```python
from build123d import *

# Parameters (mm, degrees)
CROQUIS1_R              = 20
SALIENTE_EXTRUIR1_DEPTH = 10
CROQUIS2_W              = 60
CROQUIS2_H              = 45
SALIENTE_EXTRUIR2_DEPTH = 10


with BuildPart() as part:
    # Croquis1 → Saliente-Extruir1 (new body)
    with BuildSketch(Plane.XY):
        Circle(CROQUIS1_R)
    extrude(amount=SALIENTE_EXTRUIR1_DEPTH)

    # Croquis2 → Saliente-Extruir2 (add)
    with BuildSketch(Plane.XY.offset(10)):
        Rectangle(CROQUIS2_W, CROQUIS2_H)
    extrude(amount=SALIENTE_EXTRUIR2_DEPTH)


solid = part.part
```
Model file for the job. Use its own axes, mm. A direction names the side the tool comes from. Give positions to 0.01 mm unless a question says otherwise; leave off trailing zeros. Order: outer loops, then holes, each group sorted by start corner. A loop starts at its lowest first (then second) coordinate and runs counter-clockwise, first axis right, second up.
1) Saw through at B-B, the plane x = 0. Write the cut outline in (y, z).
2) 3-axis set-ups, long thin cutter, end or side, ignore diameter. For faces 1 (the flat face through (0, -22.5, 15)), 2 (the cylindrical face through (-4.336, -19.524, 4.93)): which of +Z, -Z, +X, -X, +Y, -Y reach the whole face in a straight line?
3) Saw through at C-C, the plane z = 8. Write the cut outline in (x, y), then the cut area to 3 significant figures.
4) Wall check: probe 1 along Z at (x, y) = (13.5, -20); probe 2 along X at (y, z) = (4.5, 8); probe 3 along X at (y, z) = (16.5, 6). Give the ranges that are in metal, low to high.
5) Saw through at D-D, the plane x = 22. Write the cut outline in (y, z).
6) Pin check, flat tips, straight feed: pin 1 (1.5 mm diameter, centred on x = -16, z = 8, fed in from -Y); pin 2 (5 mm diameter, centred on x = 9, z = 6.5, fed in from -Y); pin 3 (1.5 mm diameter, centred on y = 1.5, z = 9, fed in from -X). Stop position of each tip, or through.
7) Saw through at A-A, the plane y = 0. Write the cut outline in (x, z), then the cut area to 3 significant figures.
Computed:
1. outline: (-22.5, 10) - (-20, 10) - (-20, 0) - (20, 0) - (20, 10) - (22.5, 10) - (22.5, 20) - (-22.5, 20) - close
2. face 1: +Z, -Z, +X, -X, -Y
2. face 2: -Z
3. outline: circle Ø40 at (0, 0)
3. area: 1,260 mm2
4. probe 1: z = 10 to 20
4. probe 2: x = -19.49 to 19.49
4. probe 3: x = -11.3 to 11.3
5. outline: (-22.5, 10) - (22.5, 10) - (22.5, 20) - (-22.5, 20) - close
6. pin 1: stops at y = -12.94
6. pin 2: stops at y = -18.91
6. pin 3: stops at x = -19.99
7. outline: (-30, 10) - (-20, 10) - (-20, 0) - (20, 0) - (20, 10) - (30, 10) - (30, 20) - (-30, 20) - close
7. area: 1,000 mm2
